Job drawing, mm, ordinate dimensions from the low corner. One solid piece. Round coordinates to 2 decimals unless told otherwise and drop trailing zeros. Loops run counter-clockwise (first coordinate to the right, second up) from the corner with the lowest first, then second, coordinate; pieces in that order, holes last. Notation, with made-up numbers: M -34,85 L 19,85 A25 cw 19,113 Z; hole C 64,-30.75 d4. An arc over 180 degrees is marked long. Use a Markdown table: item, result. Add a question column.
(1) Flat gauge pins, fed straight in: P1, Ø5, axis at x = 40.5, z = 39, coming from the +Y side; P2, Ø5, axis at y = 361, z = 49, coming from the -X side; P3, Ø8, axis at y = 263.5, z = 50, coming from the +X side. Where does each tip first touch, or does it go through?
(2) Wall check: L1, parallel to X at y = 590, z = 48; L2, parallel to Y at x = 100.2, z = 49.75; L3, parallel to Y at x = 112, z = 56.5. Give the ranges that are in metal, low to high.
(3) Band-saw the part on B-B, the plane x = 36.5. Write the cut outline in (y, z).
(4) Band-saw the part on A-A, the plane z = 90.5. Write the cut outline in (x, y), and give its area (3 significant figures).
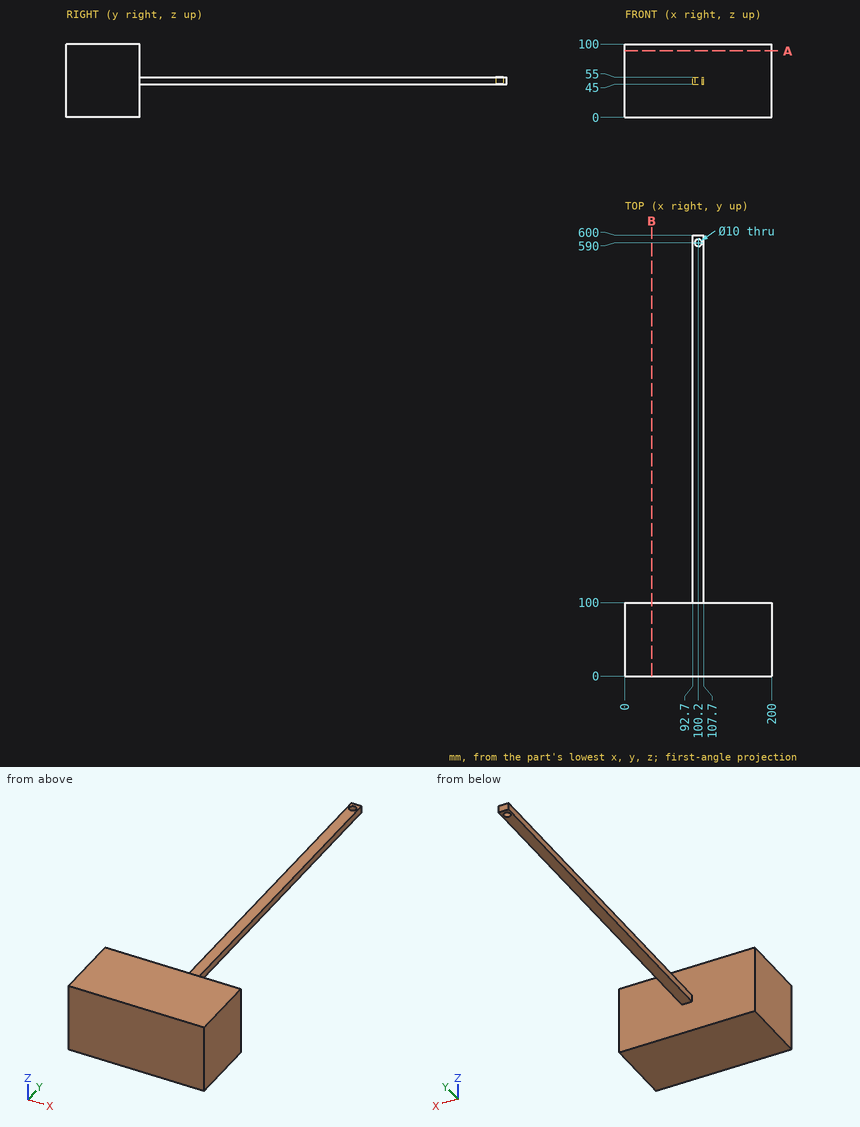
Return value:
| question | item | result |
|---|---|---|
| 1 | P1 | y = 100 |
| 1 | P2 | x = 92.7 |
| 1 | P3 | x = 107.7 |
| 2 | L1 | 92.7 to 95.2, 105.2 to 107.7 |
| 2 | L2 | 0 to 585, 595 to 600 |
| 2 | L3 | 0 to 100 |
| 3 | outline | M 0,0 L 100,0 L 100,100 L 0,100 Z |
| 4 | outline | M 0,0 L 200,0 L 200,100 L 0,100 Z |
| 4 | area | 20,000 mm^2 |
